Autodesk Inventor part; units mm, degrees
ref_plane "Work Plane1" through (0, 0, 0) normal (0, 0, -1) x (0, 1, 0)
ref_plane "YZ Plane" through (0, 0, 0) normal (1, 0, 0) x (0, 1, 0)
ref_plane "XZ Plane" through (0, 0, 0) normal (0, 1, 0) x (-1, 0, 0)
sketch "Sketch1" plane through (0, 0, 0) normal (0, 0, 1) x (1, 0, 0)
  line L0 (0, 0) -> (5, 0)
  line L1 (5, 0) -> (105, 0)
  line L2 (105, 0) -> (105, 100)
  line L3 (105, 100) -> (5, 0)
  line L4 (0, 0) -> (105, 105)
  line L5 (105, 105) -> (105, 100)
  line L6 (0, 0) -> (0, 120) construction
  dimension "d0" = 5
  dimension "d1" = 100
  dimension "d2" = 100
  dimension "d3" = 120
revolve "Revolution1" add sketch "Sketch1" angle 360 about axis through (0, 0, 0) along (0, 1, 0) contours L4 L5 L3 L0
ref_plane "Work Plane1" through (0, 0, 0) normal (0, 0, -1) x (0, 1, 0)
sketch "Sketch2" plane through (0, 0, 0) normal (0, 0, -1) x (0, 1, 0)
  line L0 (120, 0) -> (120, -10)
  line L1 (120, -10) -> (0, -10)
  line L2 (0, -10) -> (0, 0)
  line L3 (120, -10) -> (120, -110)
  line L4 (120, -110) -> (0, -110)
  line L5 (0, -110) -> (0, -10)
  line L6 (120, 0) -> (0, 0)
  dimension "d5" = 10
  dimension "d6" = 120
  dimension "d7" = 10
  dimension "d8" = 100
extrude "Extrusion1" cut sketch "Sketch2" along normal through all both and the other way through all contours L3 L4 L5 L1
extrude "Extrusion2" add sketch "Sketch2" along normal mid plane 210 contours L0 L1 L2 L6
sketch "Sketch3" plane through (0, 0, 105) normal (1, 0, 0) x (0, 0, -1)
  line L0 (0, 100) -> (100, 0)
  line L1 (0, 0) -> (0, 100)
  line L2 (100, 0) -> (0, 0)
  line L3 (110, 0) -> (210, 100)
  line L4 (210, 0) -> (110, 0)
  line L5 (210, 100) -> (210, 0)
  point P0 (105, 0)
extrude "Extrusion3" cut sketch "Sketch3" against normal through all
sketch "Sketch4" plane through (-10, 120, -105) normal (-1, 0, 0) x (0, 0, 1)
  line L0 (105, -120) -> (105, -75)
  line L1 (130, -52.5) -> (80, -52.5)
  line L2 (80, -52.5) -> (80, -97.5)
  line L3 (80, -97.5) -> (130, -97.5)
  line L4 (130, -97.5) -> (130, -52.5)
  line L5 (130, -52.5) -> (80, -97.5) construction
  line L6 (80, -52.5) -> (130, -97.5) construction
  dimension "d15" = 45
  dimension "d16" = 50
  dimension "d17" = 45
extrude "Extrusion4" cut sketch "Sketch4" against normal blind 10
sketch "Sketch5" plane through (0, 22.5, 22.5) normal (1, 0, 0) x (0, 0, -1)
  line L0 (45, 0) -> (0, 0)
  line L1 (127.5, 82.5) -> (22.5, -22.5)
  line L2 (22.5, -22.5) -> (0, 0)
extrude "Extrusion5" add sketch "Sketch5" along normal blind 25
revolve "Revolution2" cut sketch "Sketch1" angle 360 about axis through (0, 0, 0) along (0, 1, 0) contours L3 L2 L1
properties part number "Collector"
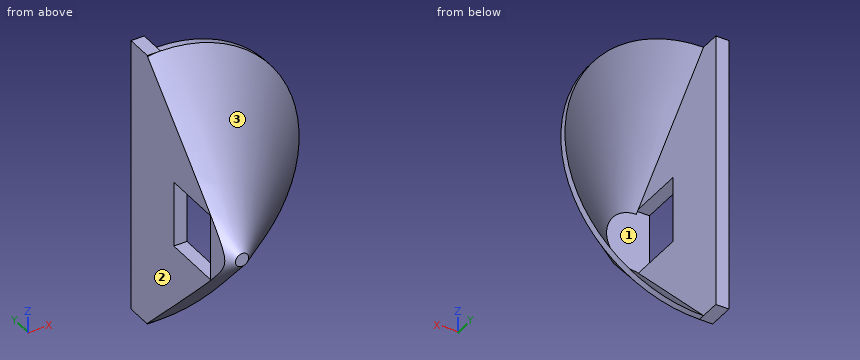
Build history of the part. All positions in model axes, mm. Face numbers are marked on the shaded views. Coordinates: 2 decimals unless noted, no trailing zeros. Order: outer loops, then holes, each group sorted by start corner. A loop starts at its lowest first (then second) coordinate and runs counter-clockwise, first axis right, second up. Notation, with made-up numbers: (-36.75, -33.75) - (20.25, -33.75) arc R22 ccw to (20.25, 1.25) - close; hole circle Ø7 at (-5.75, -38.5). An arc over 180 degrees is marked (long way). Write item = value, one per line. Start each with the question number.
1) Two-plate mould, pull along Z, no slides. Class the marked faces 1, 2 and 3: pulls with the +Z half, pulls with the -Z half, needs draft (parallel to the pull), parting line crosses it, or undercut.
2) Saw through at C-C on y = 61. Write the cut outline in (x, z), then the cut area to 3 significant figures.
3) Flat gauge pins, fed straight in: pin 1 Ø10 at (x, z) = (15.5, -25.5) entering from -Y; pin 2 Ø3 at (x, z) = (43, -62.5) entering from +Y; pin 3 Ø8 at (x, y) = (-5, 34) entering from -Z. Where does each tip first touch, or does it go through?
4) Saw through at A-A on z = 0. Write the cut outline in (x, y), then the cut area to 3 significant figures.
5) Saw through at B-B on y = 112. Write the cut outline in (x, z), then the cut area to 3 significant figures.
6) Wall check: line 1 along Z through (x, y) = (88, 104.5); line 2 along X through (y, z) = (88.5, 77); line 3 along X through (y, z) = (77.5, 13.5). Give the ranges that are in metal, low to high. Write a range as from..to.
From the geometry:
q1.face_1 = undercut
q1.face_2 = needs draft
q1.face_3 = parting line crosses it
q2.outline = (-10, -65.24) arc R66 ccw (long way) to (-10, 65.24) - (-10, 25) - (0, 25) - (0, 61) arc R61 cw to (0, -61) - (0, -25) - (-10, -25) - close
q2.area = 1,810 mm^2
q3.pin_1 = 19.84
q3.pin_2 = 77.36
q3.pin_3 = -42.73
q4.outline = (-10, 5) - (-5, 0) - (5, 0) - (105, 100) - (105, 105) - (22.5, 22.5) - (-10, 22.5) - close; (-10, 67.5) - (0, 67.5) - (0, 120) - (-10, 120) - close
q4.area = 1,500 mm^2
q5.outline = (-10, -105) - (0, -105) - (0, 105) - (-10, 105) - close
q5.area = 2,100 mm^2
q6.line_1 = -57.28..-56.36, 56.36..57.28
q6.line_2 = -10..0, 43.63..53.04
q6.line_3 = -10..0, 76.32..81.39
